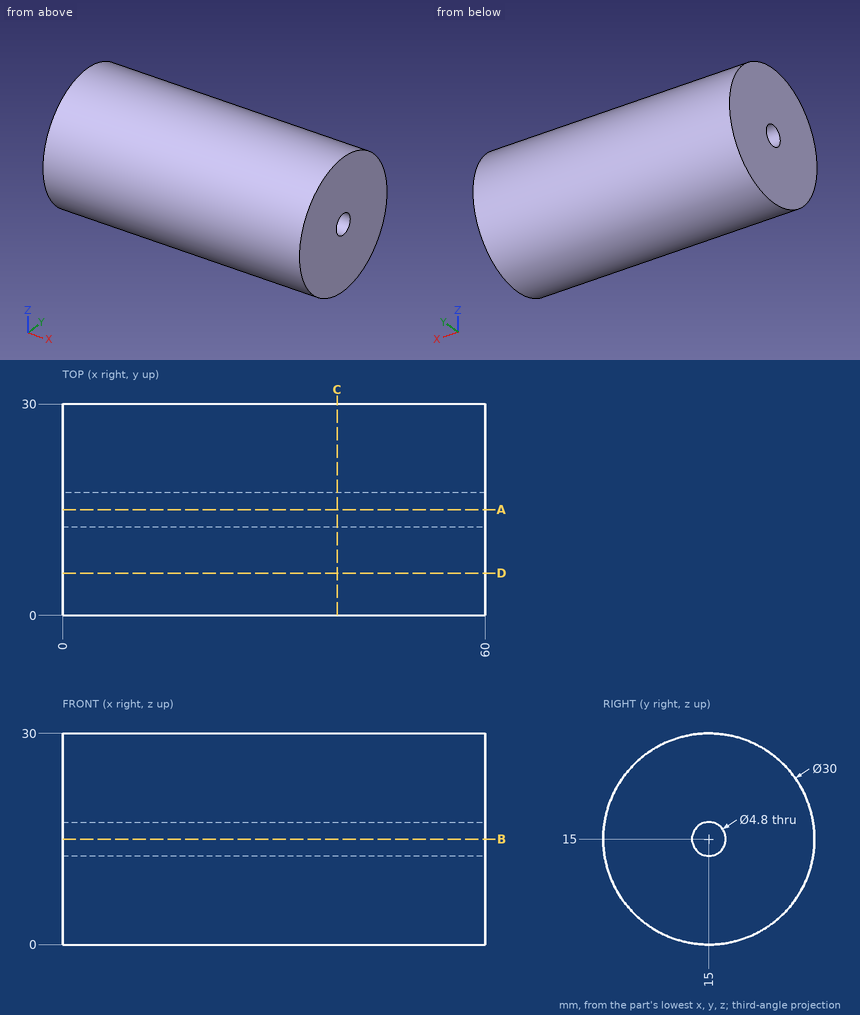
Study the drawing (mm; zero at the part's minimum x, y, z) and answer. Coordinates: 2 decimals unless noted, no trailing zeros. Loops run counter-clockwise (first coordinate to the right, second up) from the corner with the lowest first, then second, coordinate; pieces in that order, holes last. Notation, with made-up numbers: M -37,81.25 L 16,81.25 A17 ccw 16,85.25 Z; hole C 48,64.5 d4. An arc over 180 degrees is marked long. Answer in a Markdown table with one row per item. Add a question column.
1. Find section D-D, the plane y = 6. Write down the section's boundary in (x, z), then the cut area to 3 significant figures.
2. Find section A-A, the plane y = 15. Write down the section's boundary in (x, z).
3. Find section C-C, the plane x = 39. Write down the section's boundary in (y, z).
4. Flat-ended cylindrical pins translate along their axes: P1, Ø4, axis at x = 8, y = 5, coming from the -Z side; P2, Ø5, axis at x = 40, y = 24.5, coming from the -Z side; P3, Ø8, axis at x = 28, z = 21.5, coming from the -Y side. Find the tip coordinate at first contact, or state that the pin passes through.
5. Consider L1, parallel to Z at x = 31.5, y = 15; L2, parallel to Y at x = 9, z = 13; L3, parallel to Z at x = 8, y = 25.5. Determine where each line is inside the solid, lowest interval first.
Reported:
| question | item | result |
|---|---|---|
| 1 | outline | M 0,3 L 60,3 L 60,27 L 0,27 Z |
| 1 | area | 1,440 mm^2 |
| 2 | outline | M 0,0 L 60,0 L 60,12.6 L 0,12.6 Z; M 0,17.4 L 60,17.4 L 60,30 L 0,30 Z |
| 3 | outline | C 15,15 d30; hole C 15,15 d4.8 |
| 4 | P1 | stops at z = 2.31 |
| 4 | P2 | stops at z = 1.73 |
| 4 | P3 | stops at y = 0.21 |
| 5 | L1 | z = 0 to 12.6, 17.4 to 30 |
| 5 | L2 | y = 0.13 to 13.67, 16.33 to 29.87 |
| 5 | L3 | z = 4.29 to 25.71 |
